Geometry check sheet. Reference: the model listing, model coordinates, mm. Give positions to 0.01 mm unless a question says otherwise; leave off trailing zeros. Loops run counter-clockwise (first coordinate to the right, second up) from the corner with the lowest first, then second, coordinate; pieces in that order, holes last. Notation, with made-up numbers: (50, 88) -> (106, 88) arc R27 ccw to (106, 114) -> close; hole circle Ø6 at (9.5, 76). An arc over 180 degrees is marked (long way). Write each question's results on one line, items separated by ' | '. Start each with the question number.
1) Depth check by flat-ended pin: pin 1 (5 mm diameter, centred on x = 6, z = -29, fed in from -Y); pin 2 (2.5 mm diameter, centred on x = 55, z = -29, fed in from -Y); pin 3 (3 mm diameter, centred on x = 90, z = -84.95, fed in from -Y). Enter the tip coordinate at first touch or a pass-through.
2) Sectioned sample at A-A on z = -131. Record the cut outline in (x, y).
3) Scan lines: line 1 (Z direction, x = 6, y = 1.6); line 2 (Z direction, x = 90, y = 0.7); line 3 (X direction, y = 0.65, z = -25). Record each from-to range of solid material in increasing order. Write a range as from..to.
```python
from build123d import *

# Parameters (mm, degrees)
SKETCH1_W                     = 120
SKETCH1_H                     = 165
BASE_DEPTH                    = 10
PI_MOUNTHOLES_AT_2_COUNT      = 2
PI_MOUNTHOLES_AT_2_PITCH      = 49
PI_MOUNTHOLES_AT_3_COUNT      = 2
PI_MOUNTHOLES_AT_3_PITCH      = 75.927597091
PI_MOUNTHOLES_AT_4_COUNT      = 2
PI_MOUNTHOLES_AT_4_PITCH      = 58
BATTERY_MOUNTHOLES_AT_2_COUNT = 2
BATTERY_MOUNTHOLES_AT_2_PITCH = 59.95
SKETCH17_W                    = 4.7
SKETCH17_H                    = 50.5
STEPPERBRACKETSLOT_DEPTH      = 10
SKETCH18_R                    = 1.5
ANGLEBRACKET_MOUNTHOLES_DEPTH = 10


with BuildPart() as part:
    # Sketch1 → Base (new body)
    with BuildSketch(Plane(origin=(0, 0, 0), x_dir=(1, 0, 0), z_dir=(0, 1, 0))):
        with Locations((60, 82.5)):
            Rectangle(SKETCH1_W, SKETCH1_H)
    extrude(amount=BASE_DEPTH)

    # Sketch14 → Pi-MountHoles (revolve, cut)
    with BuildSketch(Plane(origin=(6, 0, -29), x_dir=(0, 0, -1), z_dir=(1, 0, 0))):
        Polygon((0, 0), (0, 10), (1.45, 10), (1.45, 2.1), (3, 2.1), (3, 0.025), (3.025, 0), align=None)
    pi_mountholes = revolve(axis=Axis((6, -6.35, -29), (0, 1, 0)), mode=Mode.SUBTRACT)

    # Pi-MountHoles at 2: Pi-MountHoles ×2
    with Locations(*[(i * PI_MOUNTHOLES_AT_2_PITCH, 0, 0) for i in range(1, PI_MOUNTHOLES_AT_2_COUNT)]):
        add(pi_mountholes, mode=Mode.SUBTRACT)

    # Pi-MountHoles at 3: Pi-MountHoles ×2
    with Locations(*[Vector(0.6453516491682099, 0, -0.7638856255460447) * (i * PI_MOUNTHOLES_AT_3_PITCH) for i in range(1, PI_MOUNTHOLES_AT_3_COUNT)]):
        add(pi_mountholes, mode=Mode.SUBTRACT)

    # Pi-MountHoles at 4: Pi-MountHoles ×2
    with Locations(*[(0, 0, -i * PI_MOUNTHOLES_AT_4_PITCH) for i in range(1, PI_MOUNTHOLES_AT_4_COUNT)]):
        add(pi_mountholes, mode=Mode.SUBTRACT)

    # Sketch16 → Battery-MountHoles (revolve, cut)
    with BuildSketch(Plane(origin=(90, 0, -25), x_dir=(0, 0, -1), z_dir=(1, 0, 0))):
        Polygon((0, 0), (0, 10), (1.1, 10), (1.1, 1.6), (2.5, 1.6), (2.5, 0.025), (2.525, 0), align=None)
    battery_mountholes = revolve(axis=Axis((90, -6.35, -25), (0, 1, 0)), mode=Mode.SUBTRACT)

    # Battery-MountHoles at 2: Battery-MountHoles ×2
    with Locations(*[(0, 0, -i * BATTERY_MOUNTHOLES_AT_2_PITCH) for i in range(1, BATTERY_MOUNTHOLES_AT_2_COUNT)]):
        add(battery_mountholes, mode=Mode.SUBTRACT)

    # Sketch17 → StepperBracketSlot (cut)
    with BuildSketch(Plane(origin=(0, 10, 0), x_dir=(1, 0, 0), z_dir=(0, 1, 0))):
        with Locations((54, 129.25)):
            Rectangle(SKETCH17_W, SKETCH17_H)
    extrude(amount=-STEPPERBRACKETSLOT_DEPTH, mode=Mode.SUBTRACT)

    # Sketch18 → AngleBracket-MountHoles (cut)
    with BuildSketch(Plane(origin=(0, 10, 0), x_dir=(1, 0, 0), z_dir=(0, 1, 0))):
        with Locations(Location((68.35, 144.75, 0), (0, 0, 270))):
            Circle(SKETCH18_R)
        with Locations(Location((68.35, 113.75, 0), (0, 0, 270))):
            Circle(SKETCH18_R)
    extrude(amount=-ANGLEBRACKET_MOUNTHOLES_DEPTH, mode=Mode.SUBTRACT)


solid = part.part
```
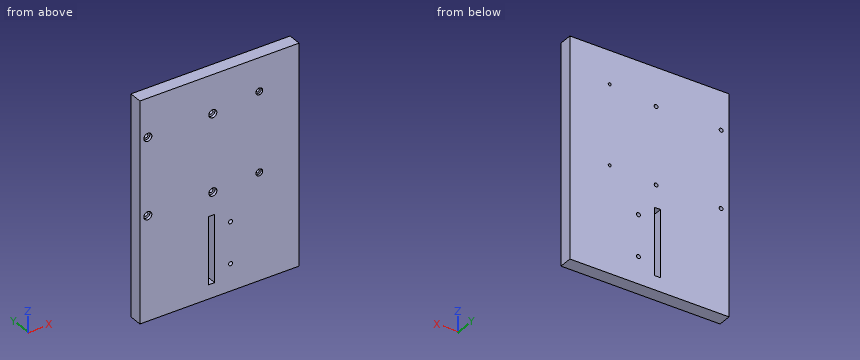
Result:
1) pin 1: y = 2.1 | pin 2: through | pin 3: y = 1.6
2) outline: (0, 0) -> (51.65, 0) -> (51.65, 10) -> (0, 10) -> close; (56.35, 0) -> (120, 0) -> (120, 10) -> (56.35, 10) -> close
3) line 1: -165..-90, -84..-32, -26..0 | line 2: -165..-87.45, -82.45..-27.5, -22.5..0 | line 3: 0..87.5, 92.5..120
